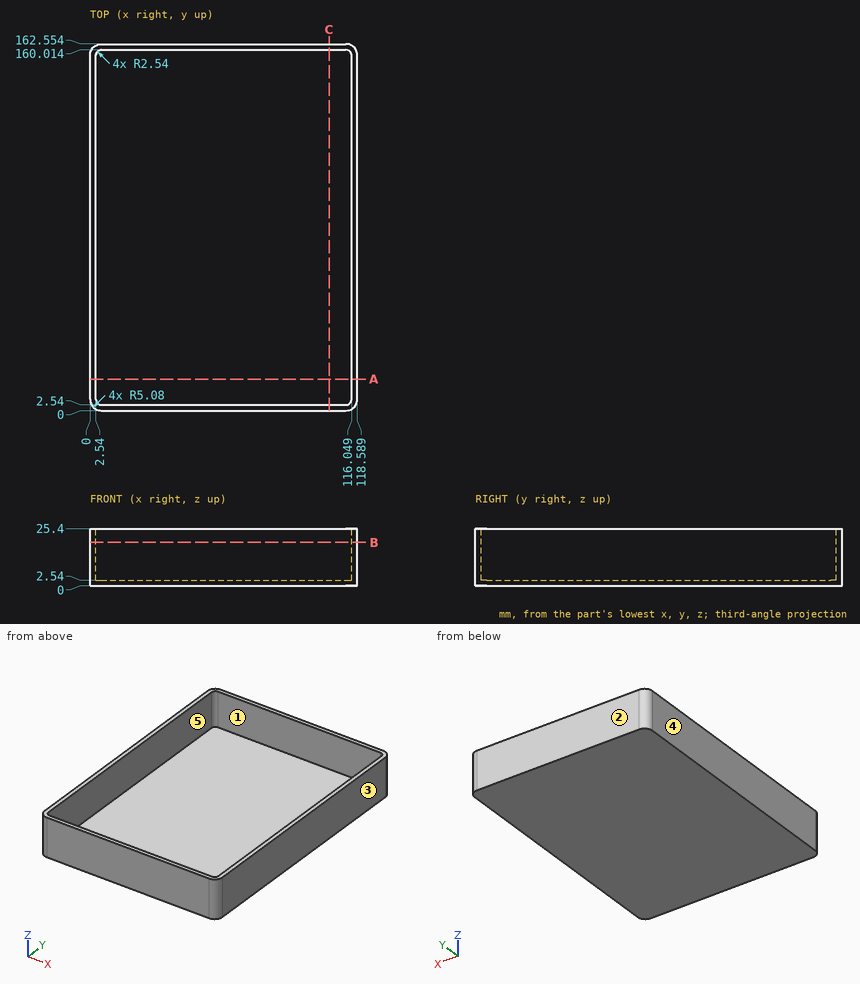
Source: three-view drawing plus pictorial views. Frame: mm from the lowest corner of the part. A direction names the side the tool comes from. Give positions to 0.01 mm unless a question says otherwise; leave off trailing zeros. Order: outer loops, then holes, each group sorted by start corner. A loop starts at its lowest first (then second) coordinate and runs counter-clockwise, first axis right, second up. Notation, with made-up numbers: (-21, -24.5) - (-10, -24.5) arc R16 ccw to (-10, -8.5) - close; hole circle Ø8 at (-26.75, 46.25). An arc over 180 degrees is marked (long way). Answer as a JSON object with one key per item and string values. Group by question number.
Q1. Cut plane A-A, the plane y = 14. Output: boundary loops of the cut face in (x, z).
Q2. Mould query, pull axis Y, two halves, no side actions, for the marked faces 1, 2 and 3. Classes: pulls with the +Y half, pulls with the -Y half, needs draft (parallel to the pull), parting line crosses it, or undercut.
Q3. Set-up query: the marked faces 4 and 5. Return all of +Z, -Z, +X, -X, +Y, -Y with unobstructed straight access to the full face (end or side cutting, diameter ignored); none if empty.
Q4. Line query: probe 1 along Y at (x, z) = (91.5, 5.25); probe 2 along X at (y, z) = (146, 21.5); probe 3 along Z at (x, y) = (77.5, 98). Output: solid intervals per line, ascending.
Q5. Cut plane B-B, the plane z = 19.25. Output: boundary loops of the cut face in (x, y), then the cut area to 3 significant figures.
Q6. First-contact query: pin 1 Ø11.5 at (x, z) = (35.5, 19.5) entering from -Y; pin 2 Ø8 at (x, y) = (36, 119) entering from +Z. Flat tips, straight axial feed; report the tip coordinate or a pass-through.
Q7. Cut plane C-C, the plane x = 106. Output: boundary loops of the cut face in (y, z), then the cut area to 3 significant figures.
Results:
{
 "1": {"outline": "(0, 0) - (118.59, 0) - (118.59, 25.4) - (116.05, 25.4) - (116.05, 2.54) - (2.54, 2.54) - (2.54, 25.4) - (0, 25.4) - close"},
 "2": {"face 1": "undercut", "face 2": "pulls with the +Y half", "face 3": "needs draft"},
 "3": {"face 4": "+Z, -Z, -X, +Y, -Y", "face 5": "+Z"},
 "4": {"probe 1": "0 to 2.54, 160.01 to 162.55", "probe 2": "0 to 2.54, 116.05 to 118.59", "probe 3": "0 to 2.54"},
 "5": {"outline": "(0, 5.08) arc R5.08 ccw to (5.08, 0) - (113.51, 0) arc R5.08 ccw to (118.59, 5.08) - (118.59, 157.47) arc R5.08 ccw to (113.51, 162.55) - (5.08, 162.55) arc R5.08 ccw to (0, 157.47) - close; hole (2.54, 5.08) arc R2.54 ccw to (5.08, 2.54) - (113.51, 2.54) arc R2.54 ccw to (116.05, 5.08) - (116.05, 157.47) arc R2.54 ccw to (113.51, 160.01) - (5.08, 160.01) arc R2.54 ccw to (2.54, 157.47) - close", "area": "1,390 mm^2"},
 "6": {"pin 1": "y = 0", "pin 2": "z = 2.54"},
 "7": {"outline": "(0, 0) - (162.55, 0) - (162.55, 25.4) - (160.01, 25.4) - (160.01, 2.54) - (2.54, 2.54) - (2.54, 25.4) - (0, 25.4) - close", "area": "529 mm^2"}
}
